Autodesk Inventor part; units mm, degrees
ref_plane "YZ Plane" through (0, 0, 0) normal (1, 0, 0) x (0, 1, 0)
ref_plane "XZ Plane" through (0, 0, 0) normal (0, 1, 0) x (-1, 0, 0)
ref_plane "XY Plane" through (0, 0, 0) normal (0, 0, 1) x (1, 0, 0)
sketch "Sketch1" plane through (0, 0, 0) normal (0, 0, 1) x (1, 0, 0)
  circle A0 centre (19.05, 19.05) radius 7.9375
  line L0 (22.7162, 25.4) -> (26.3823, 19.05)
  line L1 (26.3823, 19.05) -> (22.7162, 12.7)
  line L2 (22.7162, 12.7) -> (15.3838, 12.7)
  line L3 (15.3838, 12.7) -> (11.7177, 19.05)
  line L4 (11.7177, 19.05) -> (15.3838, 25.4)
  line L5 (15.3838, 25.4) -> (22.7162, 25.4)
  circle A1 centre (0, 19.05) radius 2.0828
  line L6 (0, 19.05) -> (19.05, 19.05) construction
  circle A2 centre (9.525, 2.5522) radius 2.0828
  circle A3 centre (28.575, 2.5522) radius 2.0828
  circle A4 centre (38.1, 19.05) radius 2.0828
  circle A5 centre (28.575, 35.5478) radius 2.0828
  circle A6 centre (9.525, 35.5478) radius 2.0828
  circle A7 centre (19.05, 19.05) radius 25.4
  line L7 (19.05, -6.35) -> (-19.05, -6.35)
  line L8 (-19.05, -6.35) -> (-19.05, 57.15)
  line L9 (6.3948, 114.3) -> (92.075, 114.3)
  line L10 (92.075, 114.3) -> (92.075, 63.5)
  line L11 (92.075, 63.5) -> (29.3317, 63.5)
  line L12 (-121.3454, 55.7276) -> (199.3502, 55.7276) construction
  arc A8 (29.3317, 63.5) -> (26.369, 43.3727) centre (29.3317, 53.2183) ccw
  circle A9 centre (85.725, 69.85) radius 2.159
  circle A10 centre (85.725, 82.55) radius 2.159
  circle A11 centre (85.725, 95.25) radius 2.159
  circle A12 centre (85.725, 107.95) radius 2.159
  line L13 (29.3317, 53.2183) -> (19.05, 53.2183) construction
  line L14 (-19.05, 57.15) -> (6.3948, 114.3)
  circle A13 centre (-12.7, 47.625) radius 2.159
  circle A14 centre (6.35, 47.625) radius 2.159
  circle A15 centre (-12.7, 22.225) radius 2.159
  circle A16 centre (12.7, 78.7335) radius 2.159
  circle A17 centre (12.7, 100.9585) radius 2.159
  point P0 (0, 0)
  point P1 (19.05, 44.45)
  dimension "d7" = 15.875
  dimension "d8" = 12.7
  dimension "d23" = 4.1656
  dimension "d25" = 19.05
  dimension "d26" = 0
  dimension "d29" = 360
  dimension "d41" = 50.8
  dimension "d42" = 19.05
  dimension "d43" = 19.05
  dimension "d44" = 38.1
  dimension "d55" = 73.025
  dimension "d57" = 4.318
  dimension "d58" = 6.35
  dimension "d59" = 6.35
  dimension "d62" = 12.7
  dimension "d67" = 6.35
  dimension "d68" = 36.6776
  dimension "d69" = 50.8
  dimension "d70" = 38.1
  dimension "d71" = 114
  dimension "d72" = 57.15
  dimension "d76" = 56.3933
  dimension "d78" = 6.35
  dimension "d79" = 9.525
  dimension "d84" = 19.05
  dimension "d91" = 31.75
  dimension "d98" = 25.4
  dimension "d105" = 22.225
  dimension "d113" = 6.35
extrude "Extrusion1" add sketch "Sketch1" along normal blind 1.27 contours A0 | A7 | A7 L7 L8 L14 L9 L10 L11 A8
sketch "Sketch2" plane through (0, 0, 1.27) normal (0, 0, 1) x (1, 0, 0)
  line L0 (-19.05, -6.35) -> (19.05, -6.35)
  arc A0 (19.05, -6.35) -> (26.369, 43.3727) centre (19.05, 19.05) ccw
  line L1 (-19.05, 57.15) -> (-19.05, -6.35)
  circle A1 centre (19.05, 19.05) radius 25.4
  line L2 (2.1167, 0.118) -> (-19.05, 19.05)
  line L3 (-19.05, 19.05) -> (-19.05, -6.35)
  line L4 (-19.05, -6.35) -> (19.05, -6.35)
  arc A2 (2.1167, 0.118) -> (19.05, -6.35) centre (19.05, 19.05) ccw
  point P0 (-19.05, 56.4751)
  point P1 (0, 0)
  dimension "d110" = 25.4
extrude "Extrusion2" cut sketch "Sketch2" against normal blind 25.4 contours L1 L2 A1 L0
fillet "Fillet2" radius 3.175 5 edges at (6.3948, 114.3, 0.635) (-19.05, 57.15, 0.635) (-19.05, 19.05, 0.635) (92.075, 63.5, 0.635) (92.075, 114.3, 0.635)
equation "\"d67\" = d58"
properties part number "Sprng Steel Arm Mount" material "Steel AISI 1080"
Can you work these out from the model? Positions are in its coordinate system, mm. A direction names the side the tool comes from. Give positions to 0.01 mm unless a question says otherwise; leave off trailing zeros. Loops run counter-clockwise (first coordinate to the right, second up) from the corner with the lowest first, then second, coordinate; pieces in that order, holes last. Notation, with made-up numbers: (77, 68.25) - (102, 68.25) arc R36 cw to (102, 106.25) - close; hole circle Ø10 at (37, 47). An arc over 180 degrees is marked (long way). One line per item, written item: value.
(1) On a 3-axis mill with a long thin cutter (end or side, diameter ignored), from which of +Z, -Z, +X, -X, +Y, -Y can I reach the whole of each face in a straight line? I mean faces 1 (the face through (91.12, 64.405, 0.644)), 2 (the face through (13.525, 22.181, 0.626)). Say none if no direction works.
Verdict:
face 1: +Z, -Z, +X, -Y
face 2: +Z, -Z
(2) If we section it at A-A, the plane y = 95.25: List the corners of the cut face in (x, z) for me (3 decimals).
Verdict:
outline: (-2.087, 0) - (83.566, 0) - (83.566, 1.27) - (-2.087, 1.27) - close; (87.884, 0) - (92.075, 0) - (92.075, 1.27) - (87.884, 1.27) - close
(3) If we mould it in two halves opening along Y, with no side actions, what happens to faces 3 (the face through (91.17, 113.345, 0.644)), 4 (the face through (-7.797, 8.985, 0.644)), 5 (the face through (5.882, 49.733, 0.626))? For each: released by +Y, released by -Y, zero draft, split by the parting line, or undercut.
Verdict:
face 3: released by +Y
face 4: released by -Y
face 5: undercut
(4) If we section it at B-B, the plane x = 0.5: List the corners of the cut face in (y, z) for me.
Verdict:
outline: (1.56, 0) - (17.03, 0) - (17.03, 1.27) - (1.56, 1.27) - close; (21.07, 0) - (101.06, 0) - (101.06, 1.27) - (21.07, 1.27) - close
(5) If we section it at C-C, the plane z = 0.7: State how many separate pieces and enclosed holes the cut face has, plus the area to 3 significant figures.
Verdict:
separate pieces: 1
enclosed holes: 16
area: 7,900 mm^2
(6) If we section it at D-D, the plane x = -12.7: List the corners of the cut face in (y, z) for me.
Verdict:
outline: (13.37, 0) - (20.07, 0) - (20.07, 1.27) - (13.37, 1.27) - close; (24.38, 0) - (45.47, 0) - (45.47, 1.27) - (24.38, 1.27) - close; (49.78, 0) - (71.41, 0) - (71.41, 1.27) - (49.78, 1.27) - close
(7) I'm going to push flat-ended pins straight in: pin 1 (5 mm diameter, centred on x = 85.725, y = 107.95, fed in from -Z); pin 2 (2.5 mm diameter, centred on x = 0, y = 19.05, fed in from +Z). Where does each tip first touch, or does it pass through?
Verdict:
pin 1: z = 0
pin 2: through
(8) I need wall thicknesses on line 1 along Y through (x, z) = (20, 1.1); line 2 along X through (y, z) = (22, 0.75); line 3 along X through (y, z) = (47, 0.4). Which ranges of each line are inside material? Lowest first, please.
Verdict:
line 1: -6.33 to 12.7, 25.4 to 48.9, 57.53 to 114.3
line 2: -19.05 to -14.85, -10.55 to 13.42, 24.68 to 44.28
line 3: -19.05 to -14.77, -10.63 to 4.28, 8.42 to 21.14
